The model under review builds one solid part; all positions refer to its coordinate system, in mm. A direction names the side the tool comes from. Round coordinates to 2 decimals unless told otherwise and drop trailing zeros. Order: outer loops, then holes, each group sorted by start corner. A loop starts at its lowest first (then second) coordinate and runs counter-clockwise, first axis right, second up. Notation, with made-up numbers: M -26,63 L -9,63 A32 cw -9,100 Z; hole C 8,-38 d7. An arc over 180 degrees is marked long. Use a Markdown table: item, result. Add a question column.
1. To check wall thickness, follow probe 1 along Y at (x, z) = (-0.5, 1.5); probe 2 along Y at (x, z) = (9, 5); probe 3 along X at (y, z) = (10, 4.75). State the ranges of each line that lie inside material, in increasing order.
2. Consider section C-C on y = 32. State the section outline as (x, z) points, then the cut area to 3 significant figures.
3. For faces 5 (the cylindrical face through (-10.747, 21.845, 3.944)), 6 (the flat face through (-9.72, -21.2, 3.94)), list the 3-axis set-ups (+Z, -Z, +X, -X, +Y, -Y) from which the entire face can be reached by the end or side of a thin tool; tool diameter is ignored.
4. Consider section B-B on z = 2.5. Count the separate pieces of the cut face and the enclosed holes in it, then the cut area to 3 significant figures.
5. Insertion check: P1, Ø3, axis at x = -28.5, z = 3, coming from the +Y side; P2, Ø4, axis at y = 32, z = 5.5, coming from the -X side; P3, Ø1.5, axis at x = 3.5, z = 7, coming from the -Y side. Each pin has a flat end and moves straight along its axis. Give the tip position at first contact, or say it passes through.
6. Consider section A-A on y = 7. State the section outline as (x, z) points, then the cut area to 3 significant figures.
7. The part is to be moulded in two halves that separate along X. For faces 1 (the flat face through (-13.5, 19, 4)), 2 (the cylindrical face through (13.7, 4.46, 3.94)), 3 (the cylindrical face through (14.073, -7.167, 3.944)), 4 (the flat face through (0, 12, 8)), say which applies: +X half, -X half, draft (parallel to the pull), parting line (faces both ways), or undercut.
8. Consider section D-D on x = -20. State the section outline as (y, z) points, then the cut area to 3 significant figures.
Autodesk Fusion 360 part; units mm, degrees
sketch "Sketch1" plane through (0, 0, 0) normal (0, 0, 1) x (1, 0, 0)
  circle A0 centre (0, 0) radius 4
  circle A1 centre (0, 0) radius 11
  line L0 (3.7528, 27.5) -> (7.5056, 34)
  line L1 (7.5056, 34) -> (3.7528, 40.5)
  line L2 (3.7528, 40.5) -> (-3.7528, 40.5)
  line L3 (-3.7528, 40.5) -> (-7.5056, 34)
  line L4 (-7.5056, 34) -> (-3.7528, 27.5)
  line L5 (-3.7528, 27.5) -> (3.7528, 27.5)
  line L6 (0, 0) -> (0, -80) construction
  circle A2 centre (0, 0) radius 48 construction
  circle A3 centre (0, 34) radius 13.5
  line L7 (-13.5, 34) -> (-13.5, 3.6173)
  arc A4 (8.2813, 23.3384) -> (9.8827, 9.8827) centre (18.6421, 17.7483) ccw
  line L8 (-22.6949, -28.6913) -> (3.6173, -13.5)
  circle A5 centre (-29.4449, -17) radius 13.5
  line L9 (-36.9504, -17) -> (-33.1976, -23.5)
  line L10 (-33.1976, -23.5) -> (-25.6921, -23.5)
  line L11 (-25.6921, -23.5) -> (-21.9393, -17)
  line L12 (-21.9393, -17) -> (-25.6921, -10.5)
  line L13 (-33.1976, -10.5) -> (-36.9504, -17)
  line L14 (-25.6921, -10.5) -> (-33.1976, -10.5)
  arc A6 (-24.3523, -4.4974) -> (-13.5, 3.6173) centre (-24.6915, 7.2704) ccw
  line L15 (36.1949, -5.3087) -> (9.8827, 9.8827)
  circle A7 centre (29.4449, -17) radius 13.5
  line L16 (33.1976, -23.5) -> (36.9504, -17)
  line L17 (36.9504, -17) -> (33.1976, -10.5)
  line L18 (33.1976, -10.5) -> (25.6921, -10.5)
  line L19 (25.6921, -10.5) -> (21.9393, -17)
  line L20 (25.6921, -23.5) -> (33.1976, -23.5)
  line L21 (21.9393, -17) -> (25.6921, -23.5)
  arc A8 (16.071, -18.841) -> (3.6173, -13.5) centre (6.0494, -25.0187) ccw
  line L22 (0, 11) -> (0, 20.5)
  line L23 (-11.5, 15.75) -> (-11.5, 20.5436)
  line L24 (-11.5, 15.75) -> (-11.5, 10.9564)
  line L25 (-9.205, 21.8156) -> (-1.5352, 17.022)
  line L26 (-1.5352, 14.478) -> (-9.205, 9.6844)
  arc A9 (-9.205, 21.8156) -> (-11.5, 20.5436) centre (-10, 20.5436) ccw
  arc A10 (-1.5352, 14.478) -> (-1.5352, 17.022) centre (-2.3302, 15.75) ccw
  arc A11 (-11.5, 10.9564) -> (-9.205, 9.6844) centre (-10, 10.9564) ccw
  arc A12 (-3.7385, -15.4375) -> (-3.7844, -12.814) centre (-4.4885, -14.1384) ccw
  line L27 (-7.8899, -17.8343) -> (-3.7385, -15.4375)
  line L28 (-7.8899, -17.8343) -> (-12.0413, -20.2311)
  arc A13 (-14.2904, -18.8796) -> (-12.0413, -20.2311) centre (-12.7913, -18.9321) ccw
  line L29 (-14.2904, -18.8796) -> (-13.9739, -9.8405)
  arc A14 (-11.7707, -8.5685) -> (-13.9739, -9.8405) centre (-12.4748, -9.893) ccw
  line L30 (-11.7707, -8.5685) -> (-3.7844, -12.814)
  arc A15 (15.2385, 4.4811) -> (12.9894, 3.1296) centre (14.4885, 3.1821) ccw
  line L31 (19.3899, 2.0843) -> (15.2385, 4.4811)
  line L32 (19.3899, 2.0843) -> (23.5413, -0.3125)
  arc A16 (23.4954, -2.936) -> (23.5413, -0.3125) centre (22.7913, -1.6116) ccw
  line L33 (23.4954, -2.936) -> (15.5091, -7.1815)
  arc A17 (13.3059, -5.9095) -> (15.5091, -7.1815) centre (14.805, -5.857) ccw
  line L34 (13.3059, -5.9095) -> (12.9894, 3.1296)
  point P0 (0, 36)
  point P1 (-11.5, 23.25)
  point P2 (-11.5, 8.25)
  point P3 (0.5, 15.75)
  dimension "d25" = 13.5
  dimension "d46" = 22
  dimension "d47" = 96
  dimension "d51" = 12
  dimension "d52" = 1.5
  dimension "d53" = 1.5
  dimension "d54" = 1.5
  dimension "d56" = 360
extrude "Extrude1" add sketch "Sketch1" along normal blind 8 contours A3 L7 A4 L8 A5 A6 L15 A7 A8 | A3 | A5 | A7 makes body 1
copy_body "Body->Comp1" bodies 1 removing the originals makes body 2 in component "Component"
component "Component" placed x (1, 0, 0) y (0, 1, 0) z (0, 0, 1) at (0, 0, 0)
Answer block:
| question | item | result |
|---|---|---|
| 1 | probe 1 | -15.88 to -10.99, 10.99 to 27.5, 40.5 to 47.49 |
| 1 | probe 2 | -13.62 to -6.32, 6.32 to 10.99, 23.94 to 44.06 |
| 1 | probe 3 | -13.5 to -11.16, -8.7 to -4.58, 4.58 to 9.78 |
| 2 | outline | M -13.5,0 L -6.35,0 L -6.35,8 L -13.5,8 Z; M 6.35,0 L 13.35,0 L 13.35,8 L 6.35,8 Z |
| 2 | area | 113 mm^2 |
| 3 | face 5 | +Z, -Z |
| 3 | face 6 | +Z, -Z, -Y |
| 4 | separate pieces | 1 |
| 4 | enclosed holes | 7 |
| 4 | area | 1,920 mm^2 |
| 5 | P1 | y = -3.5 |
| 5 | P2 | x = -13.5 |
| 5 | P3 | y = -14 |
| 6 | outline | M -13.5,0 L -8.49,0 L -8.49,8 L -13.5,8 Z; M 8.49,0 L 14.88,0 L 14.88,8 L 8.49,8 Z |
| 6 | area | 91.2 mm^2 |
| 7 | face 1 | -X half |
| 7 | face 2 | undercut |
| 7 | face 3 | undercut |
| 7 | face 4 | draft |
| 8 | outline | M -27.14,0 L -3.53,0 L -3.53,8 L -27.14,8 Z |
| 8 | area | 189 mm^2 |
